from build123d import *

# Parameters (mm, degrees)
F0_R     = 3
F1_DEPTH = 6


with BuildPart() as f1:
    # F0 (on Top) → F1 (new body)
    with BuildSketch(Plane.XY):
        with BuildLine():
            Line((-101.758, 176.250026), (-106.87925, 185.120291))
            ThreePointArc((-106.87925, 185.120291), (-185.120291, 106.87925), (-213.7585, 0))
            Line((-213.7585, 0), (-194.315, 0))
            ThreePointArc((-194.315, 0), (-168.281726, 97.1575), (-97.1575, 168.281726))
            Line((-97.1575, 168.281726), (-101.758, 176.250026))
        make_face()
        with Locations((-203.742803, 4.588549)):
            Circle(F0_R, mode=Mode.SUBTRACT)
        with Locations((-202.830195, 19.801438)):
            Circle(F0_R, mode=Mode.SUBTRACT)
        with Locations((-200.783277, 34.903588)):
            Circle(F0_R, mode=Mode.SUBTRACT)
        with Locations((-197.613498, 49.810544)):
            Circle(F0_R, mode=Mode.SUBTRACT)
        with Locations((-193.338584, 64.438938)):
            Circle(F0_R, mode=Mode.SUBTRACT)
        with Locations((-187.982442, 78.706965)):
            Circle(F0_R, mode=Mode.SUBTRACT)
        with Locations((-181.575026, 92.534829)):
            Circle(F0_R, mode=Mode.SUBTRACT)
        with Locations((-174.152169, 105.845202)):
            Circle(F0_R, mode=Mode.SUBTRACT)
        with Locations((-165.755382, 118.563645)):
            Circle(F0_R, mode=Mode.SUBTRACT)
        with Locations((-156.431624, 130.619032)):
            Circle(F0_R, mode=Mode.SUBTRACT)
        with Locations((-146.233037, 141.943945)):
            Circle(F0_R, mode=Mode.SUBTRACT)
        with Locations((-135.216656, 152.47505)):
            Circle(F0_R, mode=Mode.SUBTRACT)
        with Locations((-123.444088, 162.153452)):
            Circle(F0_R, mode=Mode.SUBTRACT)
        with BuildLine():
            ThreePointArc((-108.533127, 172.659121), (-108.122488, 171.834935), (-107.981171, 170.925026))
            ThreePointArc((-107.981171, 170.925026), (-110.187559, 168.0319), (-113.561291, 169.394347))
            ThreePointArc((-113.561291, 169.394347), (-112.74697, 173.64458), (-108.533127, 172.659121))
        make_face(mode=Mode.SUBTRACT)
        with BuildLine():
            ThreePointArc((-213.7585, 0), (0, -213.7585), (213.7585, 0))
            ThreePointArc((213.7585, 0), (106.87925, 185.120291), (-106.87925, 185.120291))
            Line((-106.87925, 185.120291), (-101.758, 176.250026))
            Line((-101.758, 176.250026), (-97.1575, 168.281726))
            ThreePointArc((-97.1575, 168.281726), (97.1575, 168.281726), (194.315, 0))
            ThreePointArc((194.315, 0), (0, -194.315), (-194.315, 0))
            Line((-194.315, 0), (-213.7585, 0))
        make_face()
        with Locations((-118.563645, -165.755382)):
            Circle(F0_R, mode=Mode.SUBTRACT)
        with Locations((-162.153452, -123.444088)):
            Circle(F0_R, mode=Mode.SUBTRACT)
        with Locations((-170.925026, -110.981171)):
            Circle(F0_R, mode=Mode.SUBTRACT)
        with Locations((-152.47505, -135.216656)):
            Circle(F0_R, mode=Mode.SUBTRACT)
        with Locations((-141.943945, -146.233037)):
            Circle(F0_R, mode=Mode.SUBTRACT)
        with Locations((-130.619032, -156.431624)):
            Circle(F0_R, mode=Mode.SUBTRACT)
        with Locations((-78.706965, -187.982442)):
            Circle(F0_R, mode=Mode.SUBTRACT)
        with Locations((-64.438938, -193.338584)):
            Circle(F0_R, mode=Mode.SUBTRACT)
        with Locations((-105.845202, -174.152169)):
            Circle(F0_R, mode=Mode.SUBTRACT)
        with Locations((-92.534829, -181.575026)):
            Circle(F0_R, mode=Mode.SUBTRACT)
        with Locations((-34.903588, -200.783277)):
            Circle(F0_R, mode=Mode.SUBTRACT)
        with Locations((-49.810544, -197.613498)):
            Circle(F0_R, mode=Mode.SUBTRACT)
        with Locations((-19.801438, -202.830195)):
            Circle(F0_R, mode=Mode.SUBTRACT)
        with Locations((-4.588549, -203.742803)):
            Circle(F0_R, mode=Mode.SUBTRACT)
        with Locations((-178.740718, -97.897601)):
            Circle(F0_R, mode=Mode.SUBTRACT)
        with Locations((-185.55682, -84.266549)):
            Circle(F0_R, mode=Mode.SUBTRACT)
        with Locations((-191.335213, -70.164244)):
            Circle(F0_R, mode=Mode.SUBTRACT)
        with Locations((-196.043581, -55.669553)):
            Circle(F0_R, mode=Mode.SUBTRACT)
        with Locations((-199.655594, -40.863534)):
            Circle(F0_R, mode=Mode.SUBTRACT)
        with Locations((-202.151052, -25.82899)):
            Circle(F0_R, mode=Mode.SUBTRACT)
        with Locations((-203.516, -10.65)):
            Circle(F0_R, mode=Mode.SUBTRACT)
        with Locations((10.65, -203.516)):
            Circle(F0_R, mode=Mode.SUBTRACT)
        with Locations((25.82899, -202.151052)):
            Circle(F0_R, mode=Mode.SUBTRACT)
        with Locations((40.863534, -199.655594)):
            Circle(F0_R, mode=Mode.SUBTRACT)
        with Locations((55.669553, -196.043581)):
            Circle(F0_R, mode=Mode.SUBTRACT)
        with Locations((70.164244, -191.335213)):
            Circle(F0_R, mode=Mode.SUBTRACT)
        with Locations((84.266549, -185.55682)):
            Circle(F0_R, mode=Mode.SUBTRACT)
        with Locations((97.897601, -178.740718)):
            Circle(F0_R, mode=Mode.SUBTRACT)
        with Locations((110.981171, -170.925026)):
            Circle(F0_R, mode=Mode.SUBTRACT)
        with Locations((123.444088, -162.153452)):
            Circle(F0_R, mode=Mode.SUBTRACT)
        with Locations((135.216656, -152.47505)):
            Circle(F0_R, mode=Mode.SUBTRACT)
        with Locations((146.233037, -141.943945)):
            Circle(F0_R, mode=Mode.SUBTRACT)
        with Locations((156.431624, -130.619032)):
            Circle(F0_R, mode=Mode.SUBTRACT)
        with Locations((165.755382, -118.563645)):
            Circle(F0_R, mode=Mode.SUBTRACT)
        with Locations((174.152169, -105.845202)):
            Circle(F0_R, mode=Mode.SUBTRACT)
        with Locations((181.575026, -92.534829)):
            Circle(F0_R, mode=Mode.SUBTRACT)
        with Locations((187.982442, -78.706965)):
            Circle(F0_R, mode=Mode.SUBTRACT)
        with Locations((193.338584, -64.438938)):
            Circle(F0_R, mode=Mode.SUBTRACT)
        with Locations((197.613498, -49.810544)):
            Circle(F0_R, mode=Mode.SUBTRACT)
        with Locations((200.783277, -34.903588)):
            Circle(F0_R, mode=Mode.SUBTRACT)
        with Locations((202.830195, -19.801438)):
            Circle(F0_R, mode=Mode.SUBTRACT)
        with Locations((203.742803, -4.588549)):
            Circle(F0_R, mode=Mode.SUBTRACT)
        with Locations((-97.897601, 178.740718)):
            Circle(F0_R, mode=Mode.SUBTRACT)
        with Locations((-84.266549, 185.55682)):
            Circle(F0_R, mode=Mode.SUBTRACT)
        with Locations((-70.164244, 191.335213)):
            Circle(F0_R, mode=Mode.SUBTRACT)
        with Locations((-55.669553, 196.043581)):
            Circle(F0_R, mode=Mode.SUBTRACT)
        with Locations((-40.863534, 199.655594)):
            Circle(F0_R, mode=Mode.SUBTRACT)
        with Locations((-25.82899, 202.151052)):
            Circle(F0_R, mode=Mode.SUBTRACT)
        with Locations((-10.65, 203.516)):
            Circle(F0_R, mode=Mode.SUBTRACT)
        with Locations((203.516, 10.65)):
            Circle(F0_R, mode=Mode.SUBTRACT)
        with Locations((202.151052, 25.82899)):
            Circle(F0_R, mode=Mode.SUBTRACT)
        with Locations((199.655594, 40.863534)):
            Circle(F0_R, mode=Mode.SUBTRACT)
        with Locations((196.043581, 55.669553)):
            Circle(F0_R, mode=Mode.SUBTRACT)
        with Locations((191.335213, 70.164244)):
            Circle(F0_R, mode=Mode.SUBTRACT)
        with Locations((185.55682, 84.266549)):
            Circle(F0_R, mode=Mode.SUBTRACT)
        with Locations((178.740718, 97.897601)):
            Circle(F0_R, mode=Mode.SUBTRACT)
        with Locations((4.588549, 203.742803)):
            Circle(F0_R, mode=Mode.SUBTRACT)
        with Locations((19.801438, 202.830195)):
            Circle(F0_R, mode=Mode.SUBTRACT)
        with Locations((49.810544, 197.613498)):
            Circle(F0_R, mode=Mode.SUBTRACT)
        with Locations((34.903588, 200.783277)):
            Circle(F0_R, mode=Mode.SUBTRACT)
        with Locations((92.534829, 181.575026)):
            Circle(F0_R, mode=Mode.SUBTRACT)
        with Locations((105.845202, 174.152169)):
            Circle(F0_R, mode=Mode.SUBTRACT)
        with Locations((64.438938, 193.338584)):
            Circle(F0_R, mode=Mode.SUBTRACT)
        with Locations((78.706965, 187.982442)):
            Circle(F0_R, mode=Mode.SUBTRACT)
        with Locations((130.619032, 156.431624)):
            Circle(F0_R, mode=Mode.SUBTRACT)
        with Locations((141.943945, 146.233037)):
            Circle(F0_R, mode=Mode.SUBTRACT)
        with Locations((152.47505, 135.216656)):
            Circle(F0_R, mode=Mode.SUBTRACT)
        with Locations((170.925026, 110.981171)):
            Circle(F0_R, mode=Mode.SUBTRACT)
        with Locations((162.153452, 123.444088)):
            Circle(F0_R, mode=Mode.SUBTRACT)
        with Locations((118.563645, 165.755382)):
            Circle(F0_R, mode=Mode.SUBTRACT)
    extrude(amount=F1_DEPTH)


solid = f1.part
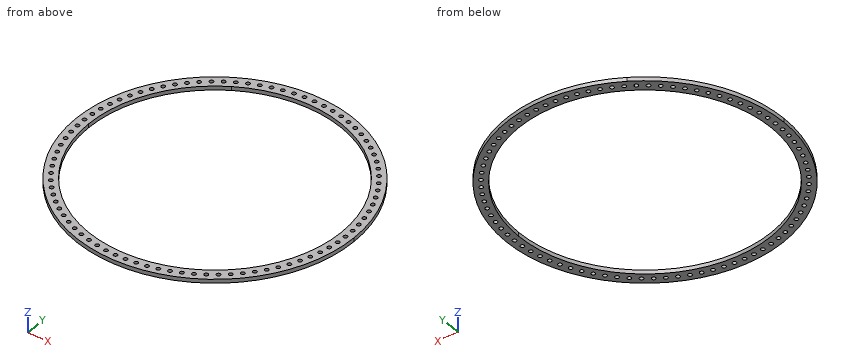
Can you work these out from the model? Positions are in its coordinate system, mm. Give positions to 0.01 mm unless a question says otherwise; leave off trailing zeros. Use one line per item in the form item = value. Start each with the question number.
Item 1: If we section it at A-A (z = 2.8): State how many separate pieces and enclosed holes the cut face has, then the cut area to 3 significant figures.
Item 2: If I drill on line 1 along Y through (x, z) = (-159, 3.35); line 2 along X through (y, z) = (-32.5, 2.6); line 3 along X through (y, z) = (-131, 3.55), over which ranges is the centre line in solid material (lowest first)?
Item 3: Will these pins go through, and if not, where does the flat tip stop? pin 1 Ø3.5 at (x, y) = (-178.74, -97.9) entering from +Z; pin 2 Ø1 at (x, z) = (-3.5, 3) entering from -Y.
Outcome:
q1.separate_pieces = 1
q1.enclosed_holes = 85
q1.area = 22,600 mm2
q2.line_1 = -142.87 to -111.7, 111.7 to 129.07, 132.17 to 142.87
q2.line_2 = -211.27 to -191.58, 191.58 to 198.99, 202.58 to 211.27
q2.line_3 = -168.91 to -143.52, 143.52 to 153.46, 159.41 to 168.91
q3.pin_1 = through
q3.pin_2 = -213.74
